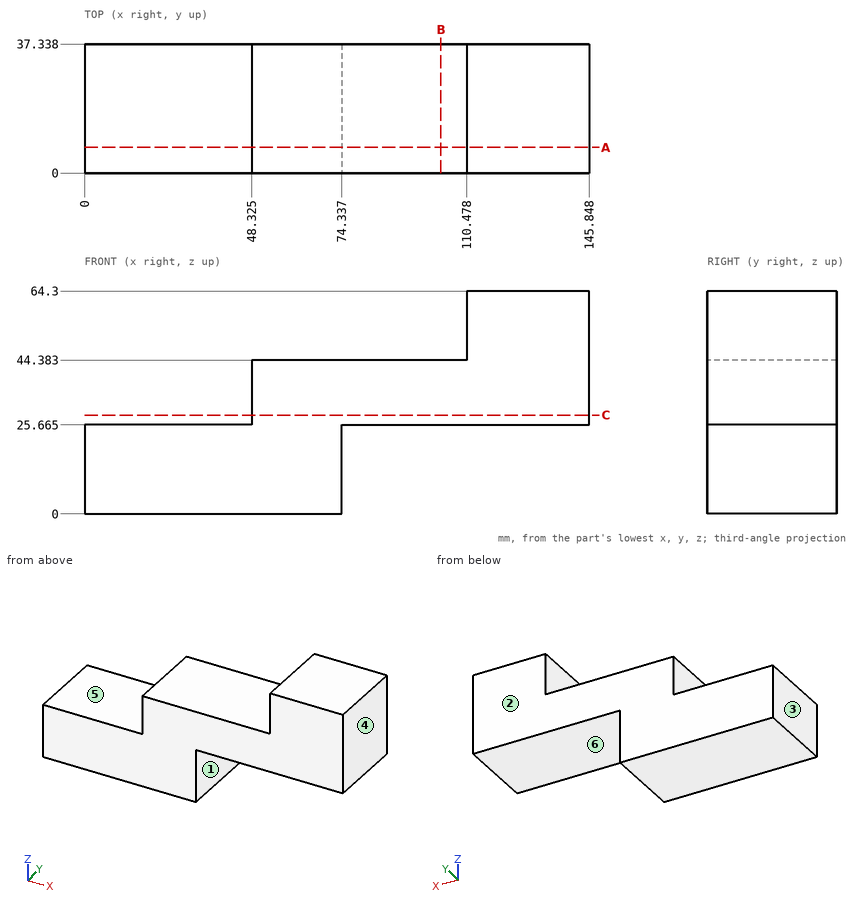
For this review, use the dimensioned drawing (mm, ordinates from the lowest corner) and the shaded views. A direction names the side the tool comes from. Give positions to 0.01 mm unless a question says otherwise; leave off trailing zeros. Write each loop counter-clockwise with the first axis right and the second up, starting at its lowest first coordinate (ties: lowest second). Pieces come first, ordered by that corner, then holes.
(1) For P1, Ø1, axis at y = 26, z = 24, coming from the +X side; P2, Ø20.5, axis at y = 21, z = 36, coming from the -X side (1 decimal); P3, Ø8, axis at x = 76, y = 12.5, coming from the +Z side, all flat-tipped, find the tip position at first contact; note any pin that passes through.
(2) To check wall thickness, follow L1, parallel to Z at x = 119, y = 13 (1 decimal); L2, parallel to Z at x = 50, y = 11.5; L3, parallel to X at y = 18.5, z = 53.5. State the ranges of each line that lie inside material, in increasing order.
(3) Consider section C-C, the plane z = 28.5. Give the boundary of the cut face in (x, y) (1 decimal), and give its area (3 significant figures).
(4) Consider section B-B, the plane x = 103. Give the boundary of the cut face in (y, z) (1 decimal).
(5) The part is to be moulded in two halves that separate along X. For the marked faces 1, 2 and 3, say which applies: released by +X, released by -X, zero draft, split by the parting line, or undercut.
(6) Consider section A-A, the plane y = 7.5. Give the boundary of the cut face in (x, z) (1 decimal), and give its area (3 significant figures).
(7) Tool access review of the marked faces 4, 5 and 6: name each direction out of +Z, -Z, +X, -X, +Y, -Y from which nothing blocks a thin tool from reaching the whole face with its end or side.
Returned:
1. P1: stops at x = 74.34
1. P2: stops at x = 48.3
1. P3: stops at z = 44.38
2. L1: z = 25.7 to 64.3
2. L2: z = 0 to 44.38
2. L3: x = 110.48 to 145.85
3. outline: (48.3, 0) - (145.8, 0) - (145.8, 37.3) - (48.3, 37.3) - close
3. area: 3,640 mm2
4. outline: (0, 25.7) - (37.3, 25.7) - (37.3, 44.4) - (0, 44.4) - close
5. face 1: released by +X
5. face 2: zero draft
5. face 3: released by -X
6. outline: (0, 0) - (74.3, 0) - (74.3, 25.7) - (145.8, 25.7) - (145.8, 64.3) - (110.5, 64.3) - (110.5, 44.4) - (48.3, 44.4) - (48.3, 25.7) - (0, 25.7) - close
6. area: 4,440 mm2
7. face 4: +Z, -Z, +X, +Y, -Y
7. face 5: +Z, -X, +Y, -Y
7. face 6: -Z, +X, +Y, -Y
